```python
from build123d import *

# Parameters (mm, degrees)
IZIM1_R                     = 9.75
IZIM1_R_2                   = 1.6
Y_KSEKLIK_EKSTR_ZYON4_DEPTH = 2.5
IZIM13_R                    = 4
Y_KSEKLIK_EKSTR_ZYON6_DEPTH = 3
IZIM14_R                    = 3
KES_EKSTR_ZYON4_DEPTH       = 4.5
IZIM15_R                    = 2
KES_EKSTR_ZYON5_DEPTH       = 2.5


with BuildPart() as part:
    # Çizim1 → Yükseklik-Ekstrüzyon4 (new body)
    with BuildSketch(Plane.XY):
        Circle(IZIM1_R)
        with Locations((-7, 0)):
            Circle(IZIM1_R_2, mode=Mode.SUBTRACT)
        with Locations((0, 7)):
            Circle(IZIM1_R_2, mode=Mode.SUBTRACT)
        with Locations((7, 0)):
            Circle(IZIM1_R_2, mode=Mode.SUBTRACT)
        with Locations((0, -7)):
            Circle(IZIM1_R_2, mode=Mode.SUBTRACT)
    extrude(amount=Y_KSEKLIK_EKSTR_ZYON4_DEPTH)

    # Çizim13 → Yükseklik-Ekstrüzyon6 (add)
    with BuildSketch(Plane(origin=(0, 0, 0), x_dir=(-1, 0, 0), z_dir=(0, 0, -1))):
        Circle(IZIM13_R)
    extrude(amount=Y_KSEKLIK_EKSTR_ZYON6_DEPTH)

    # Çizim14 → Kes-Ekstrüzyon4 (cut)
    with BuildSketch(Plane(origin=(0, 0, -3), x_dir=(-1, 0, 0), z_dir=(0, 0, -1))):
        Circle(IZIM14_R)
    extrude(amount=-KES_EKSTR_ZYON4_DEPTH, mode=Mode.SUBTRACT)

    # Çizim15 → Kes-Ekstrüzyon5 (cut)
    with BuildSketch(Plane.XY.offset(2.5)):
        Circle(IZIM15_R)
    extrude(amount=-KES_EKSTR_ZYON5_DEPTH, mode=Mode.SUBTRACT)


solid = part.part
```
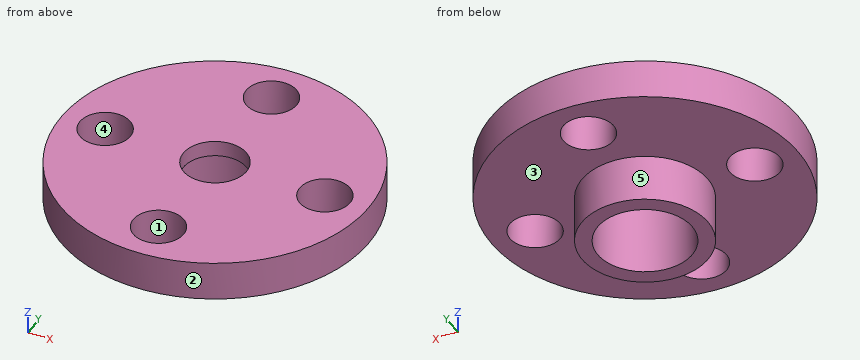
Can you work these out from the model? Positions are in its coordinate system, mm. Face numbers are marked on the shaded views. A direction names the side the tool comes from. Give positions to 0.01 mm unless a question says otherwise; leave off trailing zeros. Order: outer loops, then holes, each group sorted by start corner. A loop starts at its lowest first (then second) coordinate and runs counter-clockwise, first axis right, second up. Notation, with made-up numbers: (-35, 60.5) - (-9, 60.5) arc R15 ccw to (-9, 74.5) - close; hole circle Ø7 at (61, 58.25). An arc over 180 degrees is marked (long way). Use a Markdown table: item, result. Add a question column.
Q1. If we section it at A-A on z = 0.3: Write out the boundary of the cut face in (x, y), plus the area to 3 significant figures.
Q2. I'm going to push flat-ended pins straight in: pin 1 (1.5 mm diameter, centred on y = -1.5, z = 2, fed in from +X); pin 2 (1 mm diameter, centred on y = -6.5, z = 0.5, fed in from +X); pin 3 (1.8 mm diameter, centred on x = 1.5, y = -0.5, fed in from -Z); pin 4 (3 mm diameter, centred on x = 7, y = 0, fed in from -Z). Where does each tip first touch, or does it pass through?
Q3. If we section it at D-D on y = 1: Write out the boundary of the cut face in (x, z), plus the area to 3 significant figures.
Q4. If we mould it in two halves opening along Y, with no side actions, what happens to the marked faces 1, 2 and 3? For each: released by +Y, released by -Y, zero draft, split by the parting line, or undercut.
Q5. If we section it at C-C on x = 0: Write out the boundary of the cut face in (y, z).
Q6. If we section it at B-B on y = -7: Write out the boundary of the cut face in (x, z), plus the area to 3 significant figures.
Q7. Please list where these lines run through material, in increasing order: line 1 along Y through (x, z) = (0, 0.85); line 2 along X through (y, z) = (-0.75, 0.7); line 3 along X through (y, z) = (-1, 1.2).
Q8. On a 3-axis mill with a long thin cutter (end or side, diameter ignored), from which of +Z, -Z, +X, -X, +Y, -Y can I reach the whole of each face in a straight line? I mean the marked faces 4 and 5. Say none if no direction works.
Answers follow:
| question | item | result |
|---|---|---|
| 1 | outline | circle Ø19.5 at (0, 0); hole circle Ø3.2 at (-7, 0); hole circle Ø6 at (0, 0); hole circle Ø3.2 at (0, -7); hole circle Ø3.2 at (0, 7); hole circle Ø3.2 at (7, 0) |
| 1 | area | 238 mm^2 |
| 2 | pin 1 | stops at x = 9.72 |
| 2 | pin 2 | stops at x = 7.69 |
| 2 | pin 3 | stops at z = 1.5 |
| 2 | pin 4 | passes through |
| 3 | outline | (-9.7, 0) - (-8.25, 0) - (-8.25, 2.5) - (-9.7, 2.5) - close; (-5.75, 0) - (-3.87, 0) - (-3.87, -3) - (-2.83, -3) - (-2.83, 1.5) - (-1.73, 1.5) - (-1.73, 2.5) - (-5.75, 2.5) - close; (1.73, 1.5) - (2.83, 1.5) - (2.83, -3) - (3.87, -3) - (3.87, 0) - (5.75, 0) - (5.75, 2.5) - (1.73, 2.5) - close; (8.25, 0) - (9.7, 0) - (9.7, 2.5) - (8.25, 2.5) - close |
| 3 | area | 30.3 mm^2 |
| 4 | face 1 | undercut |
| 4 | face 2 | split by the parting line |
| 4 | face 3 | zero draft |
| 5 | outline | (-9.75, 0) - (-8.6, 0) - (-8.6, 2.5) - (-9.75, 2.5) - close; (-5.4, 0) - (-4, 0) - (-4, -3) - (-3, -3) - (-3, 1.5) - (-2, 1.5) - (-2, 2.5) - (-5.4, 2.5) - close; (2, 1.5) - (3, 1.5) - (3, -3) - (4, -3) - (4, 0) - (5.4, 0) - (5.4, 2.5) - (2, 2.5) - close; (8.6, 0) - (9.75, 0) - (9.75, 2.5) - (8.6, 2.5) - close |
| 6 | outline | (-6.79, 0) - (-1.6, 0) - (-1.6, 2.5) - (-6.79, 2.5) - close; (1.6, 0) - (6.79, 0) - (6.79, 2.5) - (1.6, 2.5) - close |
| 6 | area | 25.9 mm^2 |
| 7 | line 1 | y = -9.75 to -8.6, -5.4 to -3, 3 to 5.4, 8.6 to 9.75 |
| 7 | line 2 | x = -9.72 to -8.41, -5.59 to -2.9, 2.9 to 5.59, 8.41 to 9.72 |
| 7 | line 3 | x = -9.7 to -8.25, -5.75 to -2.83, 2.83 to 5.75, 8.25 to 9.7 |
| 8 | face 4 | +Z, -Z |
| 8 | face 5 | -Z |
